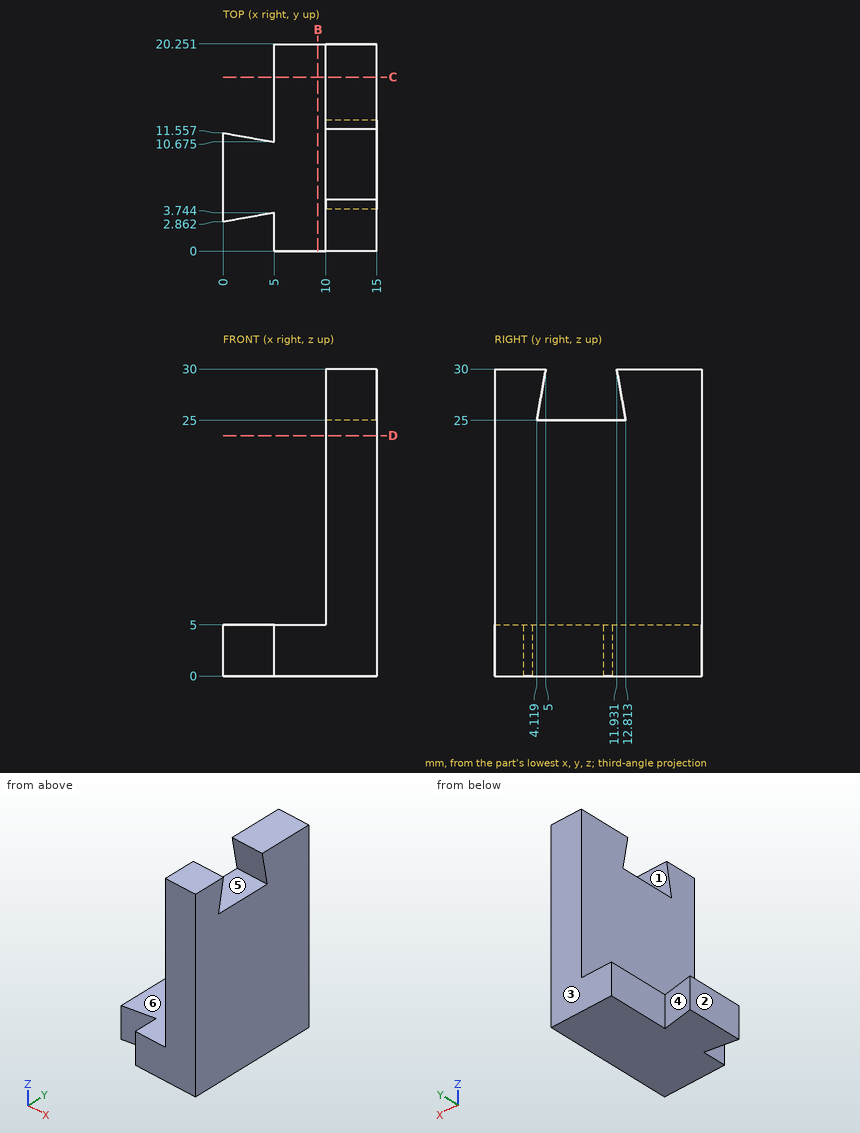
Print and shaded views of the part. All mm, measured from the part's lowest x, y and z. A direction names the side the tool comes from. Round coordinates to 2 decimals unless told otherwise and drop trailing zeros. Write each loop counter-clockwise with the first axis right and the second up, starting at its lowest first coordinate (ties: lowest second). Pieces come first, ordered by that corner, then holes. Notation, with made-up numbers: M -31,-23 L -17,-23 A23 cw -17,-9 Z; hole C 73,-29 d7. An arc over 180 degrees is marked long. Use a Markdown table: item, result. Add a question column.
1. Slice it at C-C on y = 17. Give the cut face in (x, z), then the cut area to 3 significant figures.
2. Flat gauge pins, fed straight in: P1, Ø1.5, axis at y = 17, z = 2, coming from the -X side; P2, Ø2, axis at y = 6, z = 21.5, coming from the -X side; P3, Ø1.5, axis at x = 11.5, y = 8, coming from the +Z side; P4, Ø8, axis at x = 3, z = 20, coming from the -Y side. Where does each tip first touch, or does it go through?
3. Slice it at D-D on z = 23.5. Give the cut face in (x, y).
4. Drill centre lines: probe 1 along Z at (x, y) = (1.25, 5.5); probe 2 along X at (y, z) = (2.25, 16.5); probe 3 along Y at (x, z) = (14, 26.5). Where is each one in solid material? Low to high.
5. Slice it at B-B on x = 9.25. Give the cut face in (y, z).
6. 3-axis set-ups, long thin cutter, end or side, ignore diameter. For the marked faces 4, 5 and 6: which of +Z, -Z, +X, -X, +Y, -Y reach the whole face in a straight line?
7. Pull direction Y, two halves, no side cores. Call the marked faces 1, 2 and 3: released by +Y, released by -Y, zero draft, split by the parting line, or undercut.
Reply:
| question | item | result |
|---|---|---|
| 1 | outline | M 5,0 L 15,0 L 15,30 L 10,30 L 10,5 L 5,5 Z |
| 1 | area | 175 mm^2 |
| 2 | P1 | stops at x = 5 |
| 2 | P2 | stops at x = 10 |
| 2 | P3 | stops at z = 25 |
| 2 | P4 | passes through |
| 3 | outline | M 10,0 L 15,0 L 15,20.25 L 10,20.25 Z |
| 4 | probe 1 | z = 0 to 5 |
| 4 | probe 2 | x = 10 to 15 |
| 4 | probe 3 | y = 0 to 4.38, 12.55 to 20.25 |
| 5 | outline | M 0,0 L 20.25,0 L 20.25,5 L 0,5 Z |
| 6 | face 4 | +Z, -Z, +Y |
| 6 | face 5 | +X, -X |
| 6 | face 6 | +Z, -X, +Y, -Y |
| 7 | face 1 | undercut |
| 7 | face 2 | zero draft |
| 7 | face 3 | released by +Y |
